from build123d import *

# Parameters (mm, degrees)
SKETCH_1_R             = 2
EXTRUDE_1_DEPTH        = 18
SKETCH_2_R             = 1.4
EXTRUDE_2_DEPTH        = 3
HOLE_WIZARD_M3_1_D     = 2.5
HOLE_WIZARD_M3_1_DEPTH = 7.5
HOLE_WIZARD_M3_1_TIP   = 0.751075774


with BuildPart() as part:
    # 草图1 → 凸台-拉伸1 (new body)
    with BuildSketch(Plane(origin=(0, 0, 0), x_dir=(1, 0, 0), z_dir=(0, 1, 0))):
        with Locations(Location((0, 0, 0), (0, 0, 270))):
            Circle(SKETCH_1_R)
    extrude(amount=-EXTRUDE_1_DEPTH)

    # 草图2 → 凸台-拉伸2 (add)
    with BuildSketch(Plane(origin=(0, 0, 0), x_dir=(1, 0, 0), z_dir=(0, 1, 0))):
        with Locations(Location((0, 0, 0), (0, 0, 270))):
            Circle(SKETCH_2_R)
    extrude(amount=EXTRUDE_2_DEPTH)

    # M3 螺纹孔1
    with Locations(Plane(origin=(0, -18, 0), x_dir=(0, 0, -1), z_dir=(0, -1, 0))):
        with Locations((0, 0)):
            Hole(HOLE_WIZARD_M3_1_D / 2, depth=HOLE_WIZARD_M3_1_DEPTH)
            with Locations((0, 0, -(HOLE_WIZARD_M3_1_DEPTH + HOLE_WIZARD_M3_1_TIP / 2))):  # 118° drill point
                Cone(0, HOLE_WIZARD_M3_1_D / 2, HOLE_WIZARD_M3_1_TIP, mode=Mode.SUBTRACT)


solid = part.part
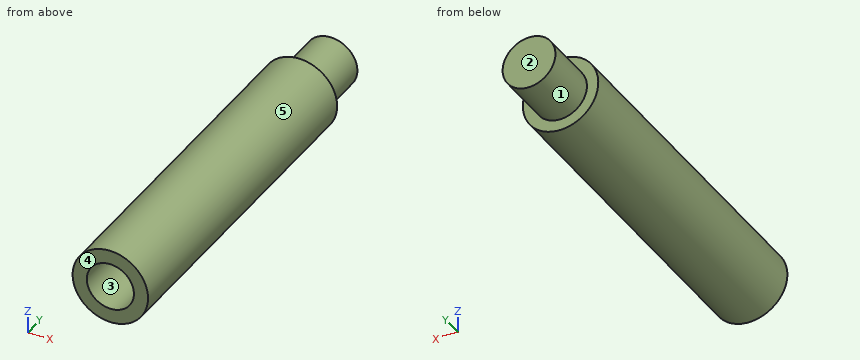
Here's how the part is built. I have some questions about the finished solid (model axes, mm). Face numbers are marked on the shaded views. A direction names the side the tool comes from. Give positions to 0.01 mm unless a question says otherwise; leave off trailing zeros. Loops run counter-clockwise (first coordinate to the right, second up) from the corner with the lowest first, then second, coordinate; pieces in that order, holes last. Notation, with made-up numbers: (66, -19.75) -> (107, -19.75) arc R6 cw to (107, -13.75) -> close; hole circle Ø11 at (-39.5, -16). An arc over 180 degrees is marked (long way). Answer as a JSON object with one key per item and string values. Group by question number.
Item 1: On a 3-axis mill with a long thin cutter (end or side, diameter ignored), from which of +Z, -Z, +X, -X, +Y, -Y can I reach the whole of each face in a straight line? I mean the marked faces 1 and 2. Say none if no direction works.
Item 2: Thinking about a two-plate mould opening in X: for the marked faces 3, 4 and 5, which applies, pulls with the +X half, pulls with the -X half, needs draft (parallel to the pull), parting line crosses it, or undercut?
Item 3: Imagine slicing it at C-C on y = -5.25. Write out the boundary of the cut face in (x, z), then the cut area to 3 significant figures.
Item 4: Will this pin go through, and if not, where does the flat tip stop? pin 1 (2 mm diameter, centred on x = 1.5, y = -10, fed in from +Z).
Item 5: I need wall thicknesses on L1, parallel to Z at x = -0.1, y = -11.5; L2, parallel to Y at x = 1.35, z = -1.1. Which ranges of each line are inside material? Lowest first, please.
Item 6: Imagine slicing it at A-A on y = 0.25. Write out the boundary of the cut face in (x, z).
Item 7: Imagine slicing it at B-B on z = -1.7. Write out the boundary of the cut face in (x, y).
Answer list:
{
 "1": {"face 1": "+Y", "face 2": "+Z, -Z, +X, -X, +Y"},
 "2": {"face 3": "undercut", "face 4": "needs draft", "face 5": "parting line crosses it"},
 "3": {"outline": "circle Ø4 at (0, 0)", "area": "12.6 mm2"},
 "4": {"pin 1": "stops at z = 1.94"},
 "5": {"L1": "z = -2 to -1.25, 1.25 to 2", "L2": "y = -18 to 0"},
 "6": {"outline": "circle Ø2.8 at (0, 0)"},
 "7": {"outline": "(-1.05, -18) -> (1.05, -18) -> (1.05, 0) -> (-1.05, 0) -> close"}
}
